Autodesk Inventor part; units mm, degrees
ref_plane "YZ Plane" through (0, 0, 0) normal (1, 0, 0) x (0, 1, 0)
ref_plane "XZ Plane" through (0, 0, 0) normal (0, 1, 0) x (-1, 0, 0)
ref_plane "XY Plane" through (0, 0, 0) normal (0, 0, 1) x (1, 0, 0)
sketch "Sketch1" plane through (0, 0, 0) normal (0, 0, 1) x (1, 0, 0)
  circle A0 centre (0, 0) radius 6
  dimension "d0" = 12
extrude "Extrusion1" add sketch "Sketch1" along normal mid plane 2
sketch "Sketch2" plane through (0, 0, -1) normal (0, 0, -1) x (-1, 0, 0)
  circle A0 centre (0, 0) radius 4
  dimension "d3" = 8
extrude "Extrusion2" add sketch "Sketch2" along normal blind 2
sketch "Sketch3" plane through (0, 0, 1) normal (0, 0, 1) x (1, 0, 0)
  circle A0 centre (0, 0) radius 3.5
  dimension "d6" = 7
extrude "Extrusion3" add sketch "Sketch3" along normal blind 1
sketch "Sketch4" plane through (0, 0, 0) normal (0, 0, 1) x (1, 0, 0)
  circle A0 centre (0, 0) radius 6
  circle A1 centre (0, 0) radius 2.1
  dimension "d9" = 4.2
extrude "Extrusion4" cut sketch "Sketch4" along normal mid plane 47 contours A1
properties part number "roller bracket" material "Steel"
Check sheet for the modelled part. Datum: model origin and axes. Units: mm. A direction names the side the tool comes from. Round coordinates to 2 decimals unless told otherwise and drop trailing zeros. Write each loop counter-clockwise with the first axis right and the second up, starting at its lowest first coordinate (ties: lowest second). Pieces come first, ordered by that corner, then holes. Notation, with made-up numbers: (39, -15) -> (72, -15) arc R12 cw to (72, -9) -> close; hole circle Ø10 at (5.5, 59.25). An arc over 180 degrees is marked (long way). Answer as CSV lines item,"result". Start each with the question number.
1) Section check D-D on y = -2.5. Enter the section's corners in (x, z).
2) Tool access check on faces 4 (the flat face through (-1.42, -3.92, -1)), 5 (the flat face through (3, -3, 1)), 6 (the flat face through (-2, -2, -3)). Record the directions out of +Z, -Z, +X, -X, +Y, -Y that give a thin tool (end or side, any length) a straight path to the whole face; none if there is none.
3) Section check C-C on z = 0.25. Enter the section's corners in (x, y), and give its area (3 significant figures).
4) Release check for a two-part mould opening along Y. For faces 1 (the cylindrical face through (2.003, -0.631, -0.535)), 2 (the cylindrical face through (0.867, 3.905, -1.986)), 3 (the flat face through (2, -2, 2)) record: pulls with the +Y half, pulls with the -Y half, needs draft (parallel to the pull), parting line crosses it, or undercut.
5) Go/stop test with a flat-tipped pin: P1, Ø3.5, axis at x = 0, y = 0, coming from the -Z side. Record where the tip stops, or that it passes through.
6) Section check A-A on x = 0. Enter the section's corners in (y, z).
7) Material ranges on line 1 (Y direction, x = 0, z = 0.7); line 2 (Z direction, x = -3.75, y = 2.5); line 3 (Y direction, x = 1.5, z = -2.45), recorded low to high. Write a range as from..to.
Found:
1,outline,"(-5.45, -1) -> (-3.12, -1) -> (-3.12, -3) -> (3.12, -3) -> (3.12, -1) -> (5.45, -1) -> (5.45, 1) -> (2.45, 1) -> (2.45, 2) -> (-2.45, 2) -> (-2.45, 1) -> (-5.45, 1) -> close"
2,face 4,"-Z"
2,face 5,"+Z"
2,face 6,"-Z, +X, -X, +Y, -Y"
3,outline,"circle Ø12 at (0, 0); hole circle Ø4.2 at (0, 0)"
3,area,"99.2 mm^2"
4,face 1,"undercut"
4,face 2,"parting line crosses it"
4,face 3,"needs draft"
5,P1,"passes through"
6,outline,"(-6, -1) -> (-4, -1) -> (-4, -3) -> (-2.1, -3) -> (-2.1, 2) -> (-3.5, 2) -> (-3.5, 1) -> (-6, 1) -> close; (2.1, -3) -> (4, -3) -> (4, -1) -> (6, -1) -> (6, 1) -> (3.5, 1) -> (3.5, 2) -> (2.1, 2) -> close"
7,line 1,"y = -6..-2.1, 2.1..6"
7,line 2,"z = -1..1"
7,line 3,"y = -3.71..-1.47, 1.47..3.71"
